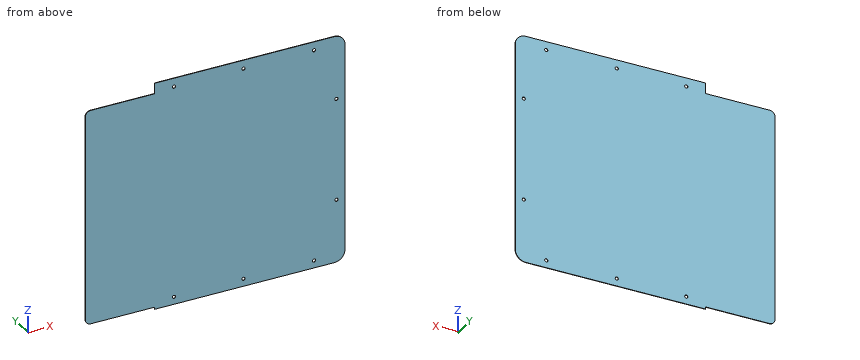
```python
from build123d import *

# Parameters (mm, degrees)
F0_R     = 1.5
F1_DEPTH = 0.5
F2_R     = 10
F3_R     = 5


with BuildPart() as f1:
    # F0 (on Front) → F1 (new body)
    with BuildSketch(Plane.XZ):
        Polygon((-178, 0), (0, 0), (0, 214), (-178, 214), (-178, 204), (-243, 204), (-243, 2), (-178, 2), align=None)
        with Locations((-160, 7)):
            Circle(F0_R, mode=Mode.SUBTRACT)
        with Locations((-95, 7)):
            Circle(F0_R, mode=Mode.SUBTRACT)
        with Locations((-29, 7)):
            Circle(F0_R, mode=Mode.SUBTRACT)
        with Locations((-8, 59)):
            Circle(F0_R, mode=Mode.SUBTRACT)
        with Locations((-160, 206)):
            Circle(F0_R, mode=Mode.SUBTRACT)
        with Locations((-8, 154.5)):
            Circle(F0_R, mode=Mode.SUBTRACT)
        with Locations((-95, 206)):
            Circle(F0_R, mode=Mode.SUBTRACT)
        with Locations((-29, 206)):
            Circle(F0_R, mode=Mode.SUBTRACT)
    extrude(amount=F1_DEPTH)

    # F2
    f2_edges = [f1.edges().sort_by_distance(p)[0] for p in [
        (0, -0.25, 214),
        (0, -0.25, 0),
    ]]
    fillet(f2_edges, radius=F2_R)

    # F3
    f3_edges = [f1.edges().sort_by_distance(p)[0] for p in [
        (-243, -0.25, 204),
        (-243, -0.25, 2),
    ]]
    fillet(f3_edges, radius=F3_R)


solid = f1.part
```
Model file for the job. Use its own axes, mm. Coordinates: 2 decimals unless noted, no trailing zeros. Order: outer loops, then holes, each group sorted by start corner. A loop starts at its lowest first (then second) coordinate and runs counter-clockwise, first axis right, second up. Notation, with made-up numbers: (50.5, 14.25) -> (70.5, 14.25) arc R9 ccw to (70.5, 25.25) -> close; hole circle Ø10 at (71.5, 2.25). An arc over 180 degrees is marked (long way). Return JSON: item names as keys, results as strings.
Item 1: Wall check: line 1 along Z through (x, y) = (-29, -0.25); line 2 along Z through (x, y) = (-8, -0.25); line 3 along Z through (x, y) = (-214.5, -0.15). Give the ranges that are in metal, low to high. Write a range as from..to.
Model answer:
{"line 1": "z = 0..5.5, 8.5..204.5, 207.5..214", "line 2": "z = 0.2..57.5, 60.5..153, 156..213.8", "line 3": "z = 2..204"}
Item 2: Slice it at B-B (x = -209). Write the cut outline in (y, z), then the cut area to 3 significant figures.
Model answer:
{"outline": "(-0.5, 2) -> (0, 2) -> (0, 204) -> (-0.5, 204) -> close", "area": "101 mm²"}
Item 3: Pin check, flat tips, straight feed: P1, Ø3.5, axis at x = -160, z = 206, coming from the +Y side; P2, Ø2.5, axis at x = -95, z = 7, coming from the -Y side. Stop position of each tip, or through.
Model answer:
{"P1": "stops at y = 0", "P2": "passes through"}
Item 4: Slice it at A-A (y = -0.35). Count the separate pieces of the cut face and the enclosed holes in it, then the cut area to 3 significant figures.
Model answer:
{"separate pieces": "1", "enclosed holes": "8", "area": "51,100 mm²"}
